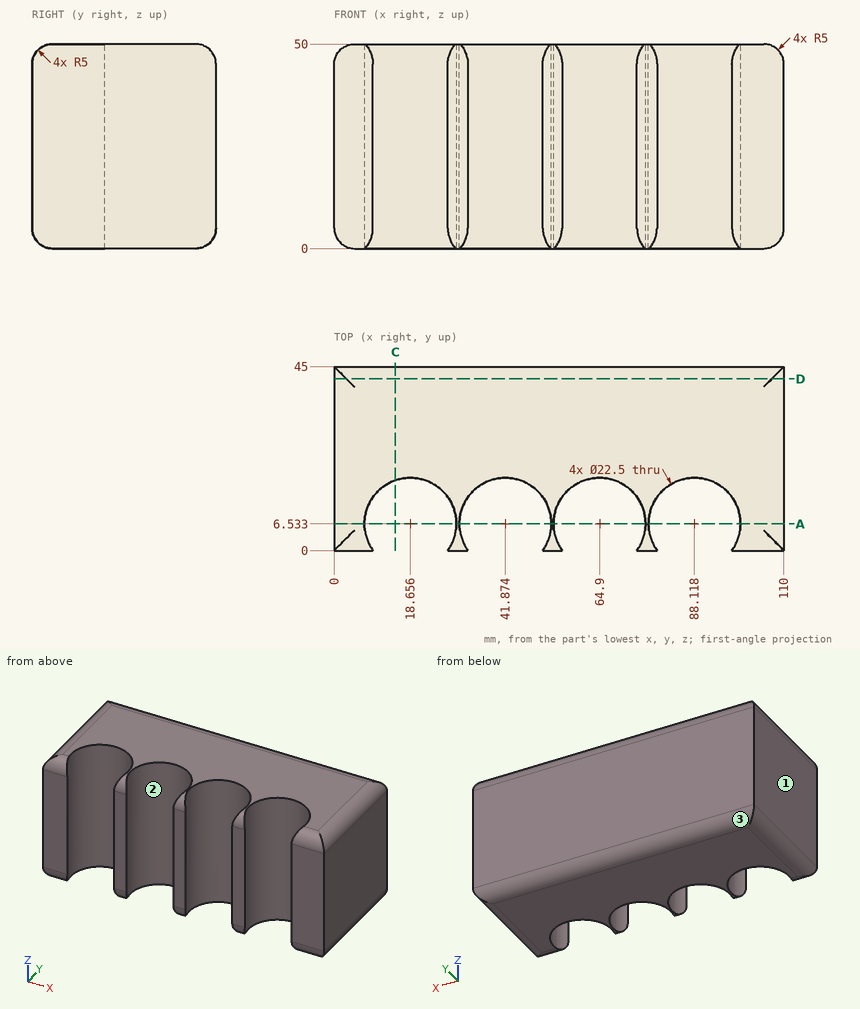
The figure shows three views and two pictorial views of one solid part (mm, origin at its lowest corner). Answer the questions. Give positions to 0.01 mm unless a question says otherwise; leave off trailing zeros. Write each loop counter-clockwise with the first axis right and the second up, starting at its lowest first coordinate (ties: lowest second). Pieces come first, ordered by that corner, then holes.
Q1. Straight lines are drawn through the part: L1, parallel to X at y = 10.5, z = 25 (1 decimal); L2, parallel to X at y = 7.5, z = 36 (1 decimal); L3, parallel to Y at x = 98.5, z = 27 (1 decimal). For each, find the intervals that lie inside material, in ascending order.
Answer:
L1: x = 0 to 8.1, 29.2 to 31.3, 52.4 to 54.4, 75.4 to 77.6, 98.6 to 110
L2: x = 0 to 7.4, 29.9 to 30.7, 53.1 to 53.7, 76.1 to 76.9, 99.3 to 110
L3: y = 0 to 2.2, 10.9 to 45
Q2. The part is cut by section A-A on y = 6.5. State how many separate pieces and enclosed holes the cut face has.
Answer:
separate pieces: 5
enclosed holes: 0
Q3. Given pin 1 (8 mm diameter, centred on x = 90.5, z = 10.5, fed in from -Y); pin 2 (18 mm diameter, centred on x = 41.87, y = 6.53, fed in from +Z); pin 3 (1 mm diameter, centred on x = 63, z = 36, fed in from -Y); pin 4 (2 mm diameter, centred on x = 40, z = 23, fed in from -Y), each flat-ended and moving along its own axis, determine where each tip first touches the part or whether it passes through.
Answer:
pin 1: stops at y = 15.8
pin 2: passes through
pin 3: stops at y = 17.52
pin 4: stops at y = 17.41
Q4. For a pull along X with two mould halves and no side action, classify the marked faces 1, 2 and 3 as released by +X, released by -X, zero draft, split by the parting line, or undercut.
Answer:
face 1: released by -X
face 2: undercut
face 3: zero draft
Q5. The part is cut by section C-C on x = 15. Give the vertices of the cut face in (y, z).
Answer:
outline: (17.17, 0) - (40, 0) arc R5 ccw to (45, 5) - (45, 45) arc R5 ccw to (40, 50) - (17.17, 50) - close
Q6. The part is cut by section D-D on y = 42. Give the vertices of the cut face in (x, z), and give its area (3 significant figures).
Answer:
outline: (0, 5) arc R5 ccw to (3, 0.42) - (107, 0.42) arc R5 ccw to (110, 5) - (110, 45) arc R5 ccw to (107, 49.58) - (3, 49.58) arc R5 ccw to (0, 45) - close
area: 5,390 mm2
